```python
from build123d import *

# Parameters (mm, degrees)
F2_W      = 21.7011459378
F2_H      = 87.9080442688
F2_W_2    = 24.2758599693
F2_H_2    = 94.1609184015
F3_DEPTH  = 30
F4_R      = 20
F5_DEPTH  = 15
F6_R      = 21
F7_DEPTH  = 30
F9_R      = 3.9
F10_DEPTH = 1.5
F11_DEPTH = 10
F13_R     = 1


with BuildPart() as f1:
    # F0 (on Front) → F1 (revolve)
    with BuildSketch(Plane.XZ):
        with BuildLine():
            Line((25, 0), (21, 0))
            ThreePointArc((21, 0), (0, -21), (-21, 0))
            Line((-21, 0), (-25, 0))
            ThreePointArc((-25, 0), (0, -25), (25, 0))
        make_face()
    revolve(axis=Axis((0, 0, 0), (1, 0, 0)))

    # F2 (on Front) → F3 (cut, symmetric)
    with BuildSketch(Plane.XZ):
        with Locations((18.8505729689, -0.3834927207)):
            Rectangle(F2_W, F2_H)
        with Locations((-20.1379299847, -2.4064816535)):
            Rectangle(F2_W_2, F2_H_2)
    extrude(amount=F3_DEPTH, both=True, mode=Mode.SUBTRACT)

    # F4 (on face) → F5 (cut)
    with BuildSketch(Plane.YZ.offset(8)):
        Circle(F4_R)
    extrude(amount=-F5_DEPTH, mode=Mode.SUBTRACT)

    # F6 (on face) → F7 (cut, symmetric)
    with BuildSketch(Plane.YZ.offset(8)):
        Circle(F6_R)
    extrude(amount=F7_DEPTH, both=True, mode=Mode.SUBTRACT)


with BuildPart() as f10:
    # F9 (on offset) → F10 (new body, symmetric)
    with BuildSketch(Plane.XZ.offset(25)):
        Circle(F9_R)
    extrude(amount=F10_DEPTH, both=True)

    # F11 (add): a face of the model
    f11_faces = [f10.faces().sort_by_distance(p)[0] for p in [
        (0, -26.5, 0),
    ]]
    extrude(f11_faces, amount=F11_DEPTH)

    # F12: union F1
    add(f1.part)

    # F13
    f13_edges = [f10.edges().sort_by_distance(p)[0] for p in [
        (-3.9, -24.693926, 0),
    ]]
    fillet(f13_edges, radius=F13_R)


solid = f10.part
```
CAD build for the part. Positions are in the model's coordinates, mm. Coordinates: 2 decimals unless noted, no trailing zeros. Write each loop counter-clockwise with the first axis right and the second up, starting at its lowest first coordinate (ties: lowest second). Pieces come first, ordered by that corner, then holes. Notation, with made-up numbers: (82.25, 70) -> (89.25, 70) arc R7 cw to (89.25, 79) -> close; hole circle Ø5 at (-37.75, 84). An arc over 180 degrees is marked (long way). Return JSON: item names as keys, results as strings. Group by question number.
Q1. Flat gauge pins, fed straight in: pin 1 (3 mm diameter, centred on x = -6, y = -22, fed in from -Z); pin 2 (1 mm diameter, centred on x = 3, y = 11.5, fed in from -Z); pin 3 (1 mm diameter, centred on x = 6, y = 0.5, fed in from +Z). Where does each tip first touch, or does it go through?
Q2. Drill centre lines: line 1 (Z direction, x = 0, y = 0); line 2 (Y direction, x = -0.25, z = 19.5); line 3 (Z direction, x = -2.5, y = -15). Where is each one in solid material? Low to high.
Q3. Pull direction Y, two halves, no side cores. Call faces 1 (the face through (0.11, 20.03, 6.31)), 2 (the face through (0, -36.5, 0)), 3 (the face through (-2.87, -30.94, 2.64)): released by +Y, released by -Y, zero draft, split by the parting line, or undercut.
Q4. Cut at A-A, the plane y = 0. Give the cut face in (x, z), then the cut area to 3 significant figures.
Q5. Cut at C-C, the plane x = 7. Give the cut face in (y, z), then the cut area to 3 significant figures.
Q6. Cut at B-B, the plane z = 10. Give the cut face in (x, y).
Q7. Cut at D-D, the plane y = -31. Give the cut face in (x, z).
Returned:
{
 "1": {"pin 1": "stops at z = -13.08", "pin 2": "stops at z = -22.26", "pin 3": "stops at z = 24.38"},
 "2": {"line 1": "z = -25 to -21, 21 to 25", "line 2": "y = -15.64 to -7.79, 7.79 to 15.64", "line 3": "z = -19.84 to -14.7, 14.7 to 19.84"},
 "3": {"face 1": "undercut", "face 2": "released by -Y", "face 3": "zero draft"},
 "4": {"outline": "(-8, -23.69) arc R25 ccw to (8, -23.69) -> (8, -21) -> (-8, -21) -> close; (-8, 21) -> (8, 21) -> (8, 23.69) arc R25 ccw to (-8, 23.69) -> close", "area": "114 mm2"},
 "5": {"outline": "circle Ø48 at (0, 0); hole circle Ø42 at (0, 0)", "area": "424 mm2"},
 "6": {"outline": "(-8, -21.47) arc R22.91 ccw to (8, -21.47) -> (8, -18.47) -> (-8, -18.47) -> close; (-8, 18.47) -> (8, 18.47) -> (8, 21.47) arc R22.91 ccw to (-8, 21.47) -> close"},
 "7": {"outline": "circle Ø7.8 at (0, 0)"}
}
